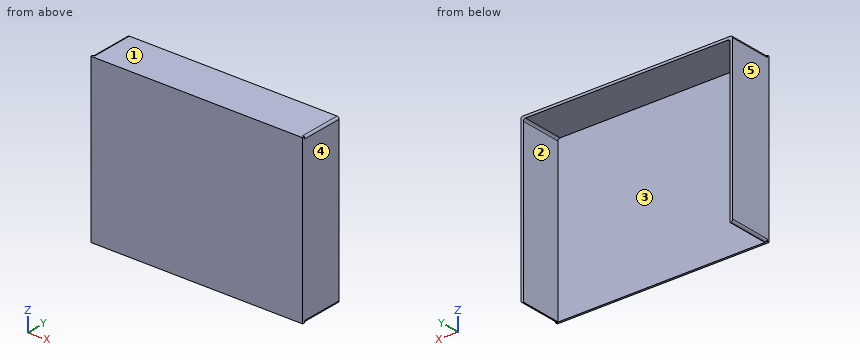
```python
from build123d import *

# Parameters (mm, degrees)
CROQUIS1_W              = 500
CROQUIS1_H              = 385
SALIENTE_EXTRUIR1_DEPTH = 5
SALIENTE_EXTRUIR2_DEPTH = 100


with BuildPart() as part:
    # Croquis1 → Saliente-Extruir1 (new body)
    with BuildSketch(Plane(origin=(0, 0, 0), x_dir=(1, 0, 0), z_dir=(0, 1, 0))):
        Rectangle(CROQUIS1_W, CROQUIS1_H)
    extrude(amount=SALIENTE_EXTRUIR1_DEPTH)

    # Croquis2 → Saliente-Extruir2 (add)
    with BuildSketch(Plane(origin=(0, 5, 0), x_dir=(1, 0, 0), z_dir=(0, 1, 0))):
        with BuildLine():
            Line((-244, 186.5), (-244, -181.5))
            ThreePointArc((-244, -181.5), (-242.535533906, -185.035533906), (-239, -186.5))
            Line((-239, -186.5), (239, -186.5))
            ThreePointArc((239, -186.5), (242.535533906, -185.035533906), (244, -181.5))
            Line((244, -181.5), (244, 186.5))
            Line((244, 186.5), (244, 192.5))
            Line((244, 192.5), (245, 192.5))
            ThreePointArc((245, 192.5), (248.535533906, 191.035533906), (250, 187.5))
            Line((250, 187.5), (250, -187.5))
            ThreePointArc((250, -187.5), (248.535533906, -191.035533906), (245, -192.5))
            Line((245, -192.5), (-245, -192.5))
            ThreePointArc((-245, -192.5), (-248.535533906, -191.035533906), (-250, -187.5))
            Line((-250, -187.5), (-250, 187.5))
            ThreePointArc((-250, 187.5), (-248.535533906, 191.035533906), (-245, 192.5))
            Line((-245, 192.5), (-244, 192.5))
            Line((-244, 192.5), (-244, 186.5))
        make_face()
    extrude(amount=SALIENTE_EXTRUIR2_DEPTH)


solid = part.part
```
Source: CAD feature listing. Evaluate the final solid. Frame: model axes, mm. Face numbers are marked on the shaded views. A direction names the side the tool comes from. Coordinates: 2 decimals unless noted, no trailing zeros. Loops run counter-clockwise (first coordinate to the right, second up) from the corner with the lowest first, then second, coordinate; pieces in that order, holes last. Notation, with made-up numbers: M 70.5,88 L 75.5,88 A31 ccw 75.5,118 Z; hole C -31.75,51 d4. An arc over 180 degrees is marked long. Use a Markdown table: item, result. Add a question column.
Q1. Section query C-C, the plane y = 59.5. Return loops of the section in (x, z), and give its area (3 significant figures).
Q2. Section query A-A, the plane z = -168. Return loops of the section in (x, y).
Q3. Section query B-B, the plane x = -201. Return loops of the section in (y, z).
Q4. First-contact query: pin 1 (1 mm diameter, centred on x = 135, y = 38.5, fed in from -Z); pin 2 (3 mm diameter, centred on x = 64, z = -67, fed in from +Y). Flat tips, straight axial feed; report the tip coordinate or a pass-through.
Q5. Material intervals for L1, parallel to X at y = 31.5, z = -3.5; L2, parallel to Y at x = -158, z = 68.5; L3, parallel to Z at x = -98, y = 83, sorted ascending.
Q6. Draft query along X for the marked faces 3, 4 and 5. Return one class per face: pulls with the +X half, pulls with the -X half, needs draft (parallel to the pull), parting line crosses it, or undercut.
Q7. Access query for the marked faces 1 and 2. Directions: +Z, -Z, +X, -X, +Y, -Y. A direction counts if a zero-diameter tool reaches every point of the face in a straight line with its end or side. Return the directions, or none.
Result:
| question | item | result |
|---|---|---|
| 1 | outline | M -250,-187.5 A5 ccw -245,-192.5 L -244,-192.5 L -244,181.5 A5 cw -239,186.5 L 239,186.5 A5 cw 244,181.5 L 244,-192.5 L 245,-192.5 A5 ccw 250,-187.5 L 250,187.5 A5 ccw 245,192.5 L -245,192.5 A5 ccw -250,187.5 Z |
| 1 | area | 7,540 mm2 |
| 2 | outline | M -250,0 L 250,0 L 250,105 L 244,105 L 244,5 L -244,5 L -244,105 L -250,105 Z |
| 3 | outline | M 0,-192.5 L 5,-192.5 L 5,186.5 L 105,186.5 L 105,192.5 L 0,192.5 Z |
| 4 | pin 1 | stops at z = 186.5 |
| 4 | pin 2 | stops at y = 5 |
| 5 | L1 | x = -250 to -244, 244 to 250 |
| 5 | L2 | y = 0 to 5 |
| 5 | L3 | z = 186.5 to 192.5 |
| 6 | face 3 | undercut |
| 6 | face 4 | pulls with the +X half |
| 6 | face 5 | pulls with the -X half |
| 7 | face 1 | +Z, +X, -X, +Y, -Y |
| 7 | face 2 | -Z, +Y |
